from build123d import *

# Parameters (mm, degrees)
F0_W     = 57.15
F0_H     = 44.45
F1_DEPTH = 25.4
F3_DEPTH = 12.7
F5_DEPTH = 25.4
F7_DEPTH = 25.4


with BuildPart() as f1:
    # F0 (on Front) → F1 (new body)
    with BuildSketch(Plane.XZ):
        with Locations((-31.7926909775, 33.1113487823)):
            Rectangle(F0_W, F0_H)
    extrude(amount=F1_DEPTH)

    # F2 (on face) → F3 (cut)
    with BuildSketch(Plane.XZ.offset(25.4)):
        Polygon((-3.2176909775, 55.3363487823), (-41.3176909775, 55.3363487823), (-15.9176909775, 10.8863487823), (-3.2176909775, 10.8863487823), align=None)
    extrude(amount=-F3_DEPTH, mode=Mode.SUBTRACT)

    # F4 (on face) → F5 (cut)
    with BuildSketch(Plane.XZ.offset(12.7)):
        with BuildLine():
            ThreePointArc((-25.4969780125, 27.6501010936), (-22.985960662, 31.6477533043), (-22.1085421056, 36.2863487823))
            ThreePointArc((-22.1085421056, 36.2863487823), (-26.8450546809, 46.1794205013), (-37.5215921901, 48.6931759045))
            Line((-37.5215921901, 48.6931759045), (-25.4969780125, 27.6501010936))
        make_face()
    extrude(amount=-F5_DEPTH, mode=Mode.SUBTRACT)

    # F6 (on face) → F7 (cut)
    with BuildSketch(Plane.XZ.offset(25.4)):
        with BuildLine():
            Line((-25.5580813343, 27.7570319068), (-37.5388390822, 48.7233579656))
            ThreePointArc((-37.5388390822, 48.7233579656), (-45.9943788824, 29.9853842652), (-25.5580813343, 27.7570319068))
        make_face()
    extrude(amount=-F7_DEPTH, mode=Mode.SUBTRACT)


solid = f1.part
Part model, mm, in its own coordinate system. A direction names the side the tool comes from. Coordinates: 2 decimals unless noted, no trailing zeros. Order: outer loops, then holes, each group sorted by start corner. A loop starts at its lowest first (then second) coordinate and runs counter-clockwise, first axis right, second up. Notation, with made-up numbers: M 4.5,59.25 L 26.5,59.25 A25 cw 26.5,86.25 Z; hole C 70.25,-24.75 d3. An arc over 180 degrees is marked long. Use a Markdown table: item, result.
(1) Cut at C-C on x = -47. Write the cut outline in (y, z), then the cut area to 3 significant figures.
A:
| item | result |
|---|---|
| outline | M -25.4,10.89 L 0,10.89 L 0,32.22 L -25.4,32.22 Z; M -25.4,40.35 L 0,40.35 L 0,55.34 L -25.4,55.34 Z |
| area | 923 mm^2 |
(2) Flat gauge pins, fed straight in: pin 1 (5 mm diameter, centred on x = -22.5, y = -20.5, fed in from +Z); pin 2 (1.5 mm diameter, centred on y = -14.5, z = 43.5, fed in from +X). Where does each tip first touch, or does it go through?
A:
| item | result |
|---|---|
| pin 1 | stops at z = 26.78 |
| pin 2 | stops at x = -44.86 |
(3) Cut at B-B on z = 41. Write the cut outline in (x, y).
A:
| item | result |
|---|---|
| outline | M -60.37,-25.4 L -46.76,-25.4 L -46.76,0 L -60.37,0 Z; M -23.02,-12.7 L -3.22,-12.7 L -3.22,0 L -23.02,0 Z |
(4) Tool access for faces 4 (the flat face through (-39, -10, 55.336)), 5 (the flat face through (-14, -12.7, 38)): list every direction of +Z, -Z, +X, -X, +Y, -Y with a clear straight run to the whole face (end or side of a thin tool).
A:
| item | result |
|---|---|
| face 4 | +Z, +X, -X, +Y, -Y |
| face 5 | +Z, +X, -Y |
(5) Cut at D-D on y = -19.5. Write the cut outline in (x, z), then the cut area to 3 significant figures.
A:
| item | result |
|---|---|
| outline | M -60.37,10.89 L -15.92,10.89 L -25.56,27.76 A12.7 cw long -37.54,48.72 L -41.32,55.34 L -60.37,55.34 Z |
| area | 1,060 mm^2 |
(6) Probe L1, parallel to Y at x = -10, z = 49; L2, parallel to X at y = -20.75, z = 36.5; L3, parallel to X at y = -6.5, z = 34. List the from-to ranges inside material, lowest first.
A:
| item | result |
|---|---|
| L1 | y = -12.7 to 0 |
| L2 | x = -60.37 to -47.67 |
| L3 | x = -60.37 to -47.46, -22.32 to -3.22 |
(7) Pull direction X, two halves, no side cores. Call faces 1 (the cylindrical face through (-46.157, -12.878, 30.279)), 2 (the flat face through (-3.218, -6, 33)), 3 (the flat face through (-48, -25.4, 28)): released by +X, released by -X, zero draft, split by the parting line, or undercut.
A:
| item | result |
|---|---|
| face 1 | undercut |
| face 2 | released by +X |
| face 3 | zero draft |
